Part model, mm, in its own coordinate system. Round coordinates to 2 decimals unless told otherwise and drop trailing zeros. Loops run counter-clockwise (first coordinate to the right, second up) from the corner with the lowest first, then second, coordinate; pieces in that order, holes last. Notation, with made-up numbers: M 1,54 L 52,54 A19 ccw 52,63 Z; hole C -9.5,-32 d4. An arc over 180 degrees is marked long. Write each question's results on one line, items separated by ' | '.
from build123d import *

# Parameters (mm, degrees)
F0_W     = 246
F0_H     = 429
F1_DEPTH = 12
F2_W     = 27
F2_H     = 224
F3_DEPTH = 25
F4_SIZE  = 11.99999
F6_D     = 3.5


# Not quite as in the source:
# - a fillet or chamfer is up to 0.001 mm smaller than in the source, because OpenCascade refuses the exact size


with BuildPart() as f1:
    # F0 (on Front) → F1 (new body)
    with BuildSketch(Plane.XZ):
        Rectangle(F0_W, F0_H)
    extrude(amount=F1_DEPTH)

    # F2 (on face) → F3 (cut)
    with BuildSketch(Plane(origin=(0, 0, 0), x_dir=(-1, 0, 0), z_dir=(0, 1, 0))):
        with Locations((-109.5, -3.5)):
            Rectangle(F2_W, F2_H)
    extrude(amount=-F3_DEPTH, mode=Mode.SUBTRACT)

    # F4 (size 12 in the source; OpenCascade refuses exactly that, so slightly less here)
    f4_edges = [f1.edges().sort_by_distance(p)[0] for p in [
        (0, 0, 214.5),
        (-123, 0, 0),
        (123, 0, 161.5),
        (123, 0, -165),
    ]]
    chamfer(f4_edges, length=F4_SIZE)

    # F6 (through all)
    with Locations(Plane.XZ.offset(12)):
        with Locations((-90.5, 195), (90.5, 195), (90.5, -156.8), (-90.5, -156.8)):
            Hole(F6_D / 2)


solid = f1.part
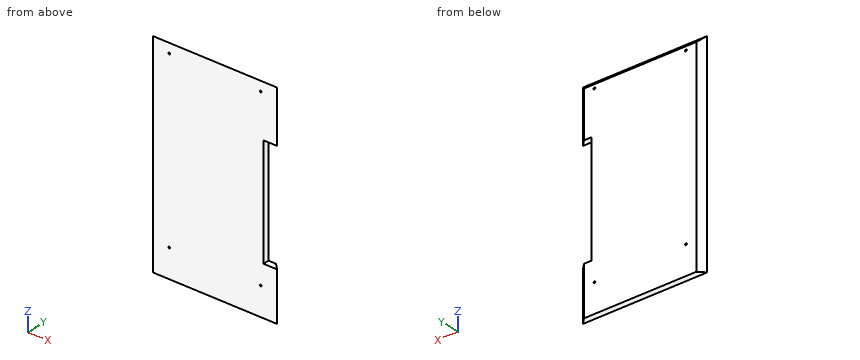
Item 1: Wall check: L1, parallel to Z at x = -90.5, y = -3.75; L2, parallel to Z at x = 90.5, y = -4.5; L3, parallel to X at y = -8.25, z = 195. Give the ranges that are in metal, low to high.
Filled sheet:
L1: -214.5 to -158.55, -155.05 to 193.25, 196.75 to 206.25 | L2: -214.5 to -158.55, -155.05 to 193.25, 196.75 to 207 | L3: -119.25 to -92.25, -88.75 to 88.75, 92.25 to 119.25
Item 2: Band-saw the part on A-A on y = -7. Give the cut face in (x, z), and give its area (3 significant figures).
Filled sheet:
outline: M -118,-214.5 L 118,-214.5 L 118,-115.5 L 96,-115.5 L 96,108.5 L 118,108.5 L 118,209.5 L -118,209.5 Z; hole C -90.5,-156.8 d3.5; hole C -90.5,195 d3.5; hole C 90.5,-156.8 d3.5; hole C 90.5,195 d3.5 | area: 95,100 mm^2
Item 3: Drop flat-ended pins along their axis: P1, Ø6, axis at y = -7, z = 13, coming from the +X side; P2, Ø1.5, axis at y = -4.5, z = -170.5, coming from the -X side; P3, Ø3, axis at x = 93.5, y = -9, coming from the +Z side. Give the stop position or say it passes through.
Filled sheet:
P1: x = 96 | P2: x = -116.25 | P3: z = 213
